```python
from build123d import *

# Parameters (mm, degrees)
BOSS_EXTRU_1_DEPTH                            = 20
TROU_POUR_TARAUDAGE_POUR_TROU_TARAUD_M3_D     = 2.5
TROU_POUR_TARAUDAGE_POUR_TROU_TARAUD_M3_DEPTH = 6
TROU_POUR_TARAUDAGE_POUR_TROU_TARAUD_M3_TIP   = 0.751075774


with BuildPart() as part:
    # Esquisse1 → Boss.-Extru.1 (new body)
    with BuildSketch(Plane(origin=(0, 0, 0), x_dir=(0, 0, -1), z_dir=(1, 0, 0))):
        Polygon((4.8, 18.9), (2.5, 18.9), (2.5, 29.8), (13.4, 29.8), (13.4, 27.5), (9.4, 27.5), (9.4, 26.5), (11.4, 24.5), (23.4, 24.5), (25.4, 26.5), (25.4, 27.5), (21.4, 27.5), (21.4, 29.8), (32.3, 29.8), (32.3, 18.9), (30, 18.9), (30, 22.9), (29, 22.9), (27, 20.9), (27, 8.9), (29, 6.9), (30, 6.9), (30, 10.9), (32.3, 10.9), (32.3, 0), (82.3, 0), (82.3, 20.480200674), (36.337333413, 59.047457256), (0, 59.047457256), (0, 0), (2.5, 0), (2.5, 10.9), (4.8, 10.9), (4.8, 6.9), (5.8, 6.9), (7.8, 8.9), (7.8, 20.9), (5.8, 22.9), (4.8, 22.9), align=None)
    extrude(amount=BOSS_EXTRU_1_DEPTH)

    # Trou pour taraudage pour trou taraudé M3x0.51
    with Locations(Plane(origin=(0, 52.543114136, -44.088907693), x_dir=(1, 0, 0), z_dir=(0, 0.7660444431189818, -0.6427876096865348))):
        with Locations((10, -5.118961569), (10, 44.881038431)):
            Hole(TROU_POUR_TARAUDAGE_POUR_TROU_TARAUD_M3_D / 2, depth=TROU_POUR_TARAUDAGE_POUR_TROU_TARAUD_M3_DEPTH)
            with Locations((0, 0, -(TROU_POUR_TARAUDAGE_POUR_TROU_TARAUD_M3_DEPTH + TROU_POUR_TARAUDAGE_POUR_TROU_TARAUD_M3_TIP / 2))):  # 118° drill point
                Cone(0, TROU_POUR_TARAUDAGE_POUR_TROU_TARAUD_M3_D / 2, TROU_POUR_TARAUDAGE_POUR_TROU_TARAUD_M3_TIP, mode=Mode.SUBTRACT)


solid = part.part
```
Design review of the part built by this model. Coordinates are the model's own, in mm. A direction names the side the tool comes from. Give positions to 0.01 mm unless a question says otherwise; leave off trailing zeros. Loops run counter-clockwise (first coordinate to the right, second up) from the corner with the lowest first, then second, coordinate; pieces in that order, holes last. Notation, with made-up numbers: (0, -17) -> (36, -17) arc R16 cw to (36, 10) -> close; hole circle Ø11 at (86.5, -15.5). An arc over 180 degrees is marked (long way). One line per item, written item: value.
Q1. We need section C-C on z = -18. Give the boundary of the cut face in (x, y), and give its area (3 significant figures).
Numbers:
outline: (0, 24.5) -> (20, 24.5) -> (20, 59.05) -> (0, 59.05) -> close
area: 691 mm^2
Q2. For L1, parallel to Z at x = 6, y = 10; L2, parallel to Z at x = 5.5, y = 3; L3, parallel to Y at x = 9, z = -31, list the stretches that pass through material, from the lowest coordinate up.
Numbers:
L1: z = -82.3 to -32.3, -30 to -27, -7.8 to -4.8, -2.5 to 0
L2: z = -82.3 to -32.3, -2.5 to 0
L3: y = 10.9 to 18.9, 29.8 to 59.05
Q3. We need section A-A on z = -31. Give the boundary of the cut face in (x, y), and give its area (3 significant figures).
Numbers:
outline: (0, 10.9) -> (20, 10.9) -> (20, 18.9) -> (0, 18.9) -> close; (0, 29.8) -> (20, 29.8) -> (20, 59.05) -> (0, 59.05) -> close
area: 745 mm^2
Q4. We need section D-D on z = -68. Give the boundary of the cut face in (x, y).
Numbers:
outline: (0, 0) -> (20, 0) -> (20, 32.48) -> (0, 32.48) -> close
Q5. Draft analysis for pull direction X (two halves, no side actions). For faces 1 (the flat face through (10, 10.9, -31)), 2 (the flat face through (20, 30, -41)), 3 (the conical face through (9.95, 18.76, -74.05)), state which applies: pulls with the +X half, pulls with the -X half, needs draft (parallel to the pull), parting line crosses it, or undercut.
Numbers:
face 1: needs draft
face 2: pulls with the +X half
face 3: undercut
Q6. For pin 1 Ø1.5 at (x, z) = (10.5, -39.5) entering from +Y; pin 2 Ø0.5 at (x, z) = (13.5, -5.5) entering from -Y; pin 3 Ø0.7 at (x, z) = (12, -3.5) entering from -Y, all flat-tipped, find the tip position at first contact; note any pin that passes through.
Numbers:
pin 1: stops at y = 57.02
pin 2: stops at y = 6.9
pin 3: stops at y = 10.9
Q7. Machinability: for faces 4 (the flat face through (10, 27.5, -23)), 5 (the flat face through (10, 10, -82.3)), 6 (the flat face through (9.9, 7.9, -28)), which of the approach directions +Z, -Z, +X, -X, +Y, -Y give a long, thin tool a straight path to every point of the face, cutting with its end or side? Answer none if there is none.
Numbers:
face 4: +X, -X
face 5: -Z, +X, -X, +Y, -Y
face 6: +X, -X, -Y
Q8. We need section B-B on y = 22. Give the number of separate pieces and of enclosed holes in the cut face, and give its area (3 significant figures).
Numbers:
separate pieces: 4
enclosed holes: 1
area: 1,080 mm^2
